from build123d import *

# Parameters (mm, degrees)
SKETCH1_W            = 218.44
SKETCH1_H            = 190.5
BOSS_EXTRUDE1_DEPTH  = 31.75
SKETCH2_W            = 206.375
SKETCH2_H            = 180.975
CUT_EXTRUDE1_DEPTH   = 149.356440373
SKETCH3_R            = 4.8895
CUT_EXTRUDE2_DEPTH   = 241.409356307
SKETCH4_W            = 12.7
SKETCH4_H            = 12.7
BOSS_EXTRUDE2_DEPTH  = 31.75
SKETCH5_R            = 1.27
CUT_EXTRUDE3_DEPTH   = 157.81286108
FILLET1_R            = 6.35
SKETCH6_W            = 12.7
SKETCH6_H            = 12.7
SKETCH6_R            = 1.27
BOSS_EXTRUDE3_DEPTH  = 31.75
FILLET4_R            = 6.35
FILLET1_OF_MIRROR8_R = 6.35
FILLET4_OF_MIRROR8_R = 6.35
FILLET5_R            = 2.54


with BuildPart() as part:
    # Sketch1 → Boss-Extrude1 (new body)
    with BuildSketch(Plane.XY):
        Rectangle(SKETCH1_W, SKETCH1_H)
    extrude(amount=BOSS_EXTRUDE1_DEPTH)

    # Sketch2 → Cut-Extrude1 (cut, through all)
    with BuildSketch(Plane.XY.offset(31.75)):
        Rectangle(SKETCH2_W, SKETCH2_H)
    extrude(amount=-CUT_EXTRUDE1_DEPTH, mode=Mode.SUBTRACT)

    # Sketch3 → Cut-Extrude2 (cut, through all)
    with BuildSketch(Plane(origin=(109.22, 0, 0), x_dir=(0, 0, -1), z_dir=(1, 0, 0))):
        Circle(SKETCH3_R)
        with Locations((0, 57.404)):
            Circle(SKETCH3_R)
        with Locations((0, -57.404)):
            Circle(SKETCH3_R)
    extrude(amount=-CUT_EXTRUDE2_DEPTH, mode=Mode.SUBTRACT)

    # Sketch4 → Boss-Extrude2 (add, through all)
    with BuildSketch(Plane(origin=(0, 0, 0), x_dir=(-1, 0, 0), z_dir=(0, 0, -1))):
        with Locations((-102.87, 101.6)):
            Rectangle(SKETCH4_W, SKETCH4_H)
    boss_extrude2 = extrude(amount=-BOSS_EXTRUDE2_DEPTH)

    # Sketch5 → Cut-Extrude3 (cut, through all)
    with BuildSketch(Plane.XY.offset(31.75)):
        with Locations((102.87, 101.6)):
            Circle(SKETCH5_R)
    cut_extrude3 = extrude(amount=-CUT_EXTRUDE3_DEPTH, mode=Mode.SUBTRACT)

    # Fillet1
    fillet1_edges = [part.edges().sort_by_distance(p)[0] for p in [
        (96.52, 107.95, 15.875),
        (109.22, 107.95, 15.875),
    ]]
    fillet(fillet1_edges, radius=FILLET1_R - 0.0001)  # a hair under: the kernel refuses the full size

    # Sketch6 → Boss-Extrude3 (add, through all)
    with BuildSketch(Plane(origin=(0, 0, 0), x_dir=(-1, 0, 0), z_dir=(0, 0, -1))):
        with Locations((-102.87, -101.6)):
            Rectangle(SKETCH6_W, SKETCH6_H)
        with Locations((-102.87, -101.6)):
            Circle(SKETCH6_R, mode=Mode.SUBTRACT)
    boss_extrude3 = extrude(amount=-BOSS_EXTRUDE3_DEPTH)

    # Fillet4
    fillet4_edges = [part.edges().sort_by_distance(p)[0] for p in [
        (109.22, -107.95, 15.875),
        (96.52, -107.95, 15.875),
    ]]
    fillet(fillet4_edges, radius=FILLET4_R - 0.0001)  # a hair under: the kernel refuses the full size

    # Mirror8: Boss-Extrude2, Cut-Extrude3, Boss-Extrude3 across plane
    add(boss_extrude2.mirror(Plane(origin=(0, 0, 0), x_dir=(0, 0, 1), z_dir=(1, 0, 0))))
    add(cut_extrude3.mirror(Plane(origin=(0, 0, 0), x_dir=(0, 0, 1), z_dir=(1, 0, 0))), mode=Mode.SUBTRACT)
    add(boss_extrude3.mirror(Plane(origin=(0, 0, 0), x_dir=(0, 0, 1), z_dir=(1, 0, 0))))

    # Fillet1 of Mirror8
    fillet1_of_mirror8_edges = [part.edges().sort_by_distance(p)[0] for p in [
        (-96.52, 107.95, 15.875),
        (-109.22, 107.95, 15.875),
    ]]
    fillet(fillet1_of_mirror8_edges, radius=FILLET1_OF_MIRROR8_R - 0.0001)  # a hair under: the kernel refuses the full size

    # Fillet4 of Mirror8
    fillet4_of_mirror8_edges = [part.edges().sort_by_distance(p)[0] for p in [
        (-109.22, -107.95, 15.875),
        (-96.52, -107.95, 15.875),
    ]]
    fillet(fillet4_of_mirror8_edges, radius=FILLET4_OF_MIRROR8_R - 0.0001)  # a hair under: the kernel refuses the full size

    # Fillet5
    fillet5_edges = [part.edges().sort_by_distance(p)[0] for p in [
        (96.52, -95.25, 15.875),
        (-96.52, 95.25, 15.875),
        (-96.52, -95.25, 15.875),
        (96.52, 95.25, 15.875),
    ]]
    fillet(fillet5_edges, radius=FILLET5_R)


solid = part.part
Part model, mm, in its own coordinate system. A direction names the side the tool comes from. Round coordinates to 2 decimals unless told otherwise and drop trailing zeros. Write each loop counter-clockwise with the first axis right and the second up, starting at its lowest first coordinate (ties: lowest second). Pieces come first, ordered by that corner, then holes. Notation, with made-up numbers: M -16.5,35.25 L -0.5,35.25 A20 ccw -0.5,74.25 Z; hole C -35,63 d10. An arc over 180 degrees is marked long. Return JSON: item names as keys, results as strings. Group by question number.
(1) Saw through at A-A on x = -36. Write the cut outline in (y, z).
(2) Drill centre lines: probe 1 along X at (y, z) = (-101.6, 16); probe 2 along Y at (x, z) = (102.87, 11); probe 3 along X at (y, z) = (-77.5, 2). Where is each one in solid material? Low to high.
(3) Two-plate mould, pull along Y, no slides. Class faces 1 (the face through (-106, 1, 31.75)), 2 (the face through (-1, 90.488, 16)), 3 (the face through (-107.41, -106.04, 16.1)): +Y half, -Y half, draft (parallel to the pull), parting line (faces both ways), or undercut.
(4) Pin check, flat tips, straight feed: pin 1 Ø16 at (x, z) = (51, 23) entering from -Y; pin 2 Ø2 at (x, y) = (102.87, -101.6) entering from +Z; pin 3 Ø16 at (x, z) = (29, 8.5) entering from +Y. Stop position of each tip, or through.
(5) Saw through at B-B on z = 28.5. Count the separate pieces of the cut face and the enclosed holes in it, then the cut area to 3 significant figures.
(6) Saw through at C-C on y = 0. Write the cut outline in (x, z).
(7) Which spindle directions (+Z, -Z, +X, -X, +Y, -Y) get a long thin tool onto all of the face, cutting with end or side? Do faces 4 (the face through (-98.33, 106.04, 16.1)), 5 (the face through (-103.188, -1, 16)), 6 (the face through (-98.43, -106.14, 16.1)). Say none if no direction does.
Returned:
{
 "1": {"outline": "M -95.25,0 L -90.49,0 L -90.49,31.75 L -95.25,31.75 Z; M 90.49,0 L 95.25,0 L 95.25,31.75 L 90.49,31.75 Z"},
 "2": {"probe 1": "-109.22 to -104.14, -101.6 to -96.52, 96.52 to 101.6, 104.14 to 109.22", "probe 2": "-107.95 to -102.87, -100.33 to -90.49, 90.49 to 100.33, 102.87 to 107.95", "probe 3": "-109.22 to -103.19, 103.19 to 109.22"},
 "3": {"face 1": "draft", "face 2": "undercut", "face 3": "-Y half"},
 "4": {"pin 1": "y = -95.25", "pin 2": "through", "pin 3": "y = 95.25"},
 "5": {"separate pieces": "1", "enclosed holes": "5", "area": "4,830 mm²"},
 "6": {"outline": "M -109.22,4.89 L -103.19,4.89 L -103.19,31.75 L -109.22,31.75 Z; M 103.19,4.89 L 109.22,4.89 L 109.22,31.75 L 103.19,31.75 Z"},
 "7": {"face 4": "+Z, -Z, +Y", "face 5": "+Z, -Z", "face 6": "+Z, -Z, -Y"}
}
